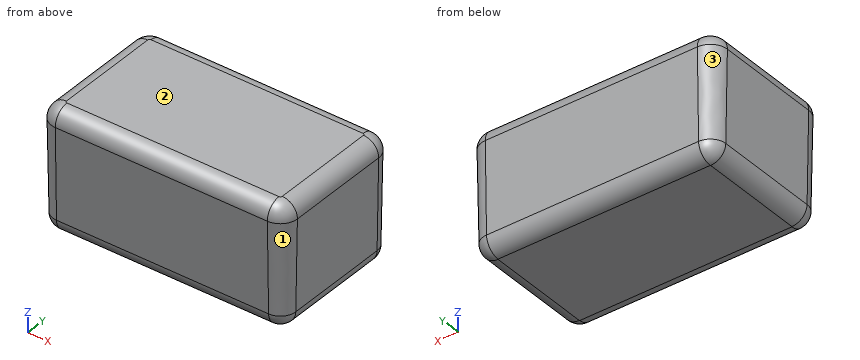
```python
from build123d import *

# Parameters (mm, degrees)
BOSS_EXTRUDE1_DEPTH = 80
DRAFT1_ANGLE        = 1
FILLET1_R           = 10
SHELL2_T            = 2.5


with BuildPart() as part:
    # Sketch1 → Boss-Extrude1 (new body)
    with BuildSketch(Plane.XY):
        with BuildLine():
            Line((-70, 45), (70, 45))
            ThreePointArc((70, 45), (77.071067812, 42.071067812), (80, 35))
            Line((80, 35), (80, -35))
            ThreePointArc((80, -35), (77.071067812, -42.071067812), (70, -45))
            Line((70, -45), (-70, -45))
            ThreePointArc((-70, -45), (-77.071067812, -42.071067812), (-80, -35))
            Line((-80, -35), (-80, 35))
            ThreePointArc((-80, 35), (-77.071067812, 42.071067812), (-70, 45))
        make_face()
    extrude(amount=BOSS_EXTRUDE1_DEPTH)

    # Draft1
    draft1_faces = [part.faces().sort_by_distance(p)[0] for p in [
        (-77.071067812, -42.071067812, 40),
        (-77.071067812, 42.071067812, 40),
        (77.071067812, 42.071067812, 40),
        (77.071067812, -42.071067812, 40),
        (80, 0, 40),
        (0, -45, 40),
        (-80, 0, 40),
        (0, 45, 40),
    ]]
    draft(draft1_faces, Plane(origin=(-70, 35, 0), x_dir=(-1, 0, 0), z_dir=(0, 0, -1)), DRAFT1_ANGLE)

    # Fillet1
    fillet1_edges = [part.edges().sort_by_distance(p)[0] for p in [
        (0, -45, 0),
        (-77.071067812, -42.071067812, 0),
        (-80, 0, 0),
        (-77.071067812, 42.071067812, 0),
        (-78.058475394, -43.058475394, 80),
        (0, -46.396405194, 80),
        (78.058475394, -43.058475394, 80),
        (81.396405194, 0, 80),
        (78.058475394, 43.058475394, 80),
        (0, 46.396405194, 80),
        (-78.058475394, 43.058475394, 80),
        (0, 45, 0),
        (-81.396405194, 0, 80),
        (77.071067812, 42.071067812, 0),
        (80, 0, 0),
        (77.071067812, -42.071067812, 0),
    ]]
    fillet(fillet1_edges, radius=FILLET1_R)

    # Shell2 (no face opened: a closed hollow body)
    add(offset(amount=-SHELL2_T, mode=Mode.PRIVATE), mode=Mode.SUBTRACT)


solid = part.part
```
Geometry: final body of the model. Coordinates: model frame, mm. Face numbers are marked on the shaded views. A direction names the side the tool comes from. Round coordinates to 2 decimals unless told otherwise and drop trailing zeros. Write each loop counter-clockwise with the first axis right and the second up, starting at its lowest first coordinate (ties: lowest second). Pieces come first, ordered by that corner, then holes.
Item 1: Section query B-B (y = -9). Return loops of the section in (x, z).
Item 2: Pin query (flat end, axial travel): P1, Ø4, axis at x = -23.5, z = 45, coming from the +Y side; P2, Ø8, axis at x = -9.5, z = 26, coming from the -Y side; P3, Ø5, axis at y = 30.5, z = 25, coming from the -X side. Return the tip coordinate at first contact, or that it passes through.
Item 3: Set-up query: the marked faces 1, 2 and 3. Return all of +Z, -Z, +X, -X, +Y, -Y with unobstructed straight access to the full face (end or side cutting, diameter ignored); none if empty.
Item 4: Material intervals for L1, parallel to X at y = 2, z = 68; L2, parallel to Z at x = -2, y = -14; L3, parallel to Y at x = 36.5, z = 68, sorted ascending.
Item 5: Section query A-A (x = 61). Return loops of the section in (y, z), plus the area to 3 significant figures.
Completed:
1. outline: (-81.22, 69.83) - (-80.17, 9.83) arc R10 ccw to (-70.17, 0) - (70.17, 0) arc R10 ccw to (80.17, 9.83) - (81.22, 69.83) arc R10 ccw to (71.22, 80) - (-71.22, 80) arc R10 ccw to start; hole (-78.72, 69.87) - (-77.67, 9.87) arc R7.5 ccw to (-70.17, 2.5) - (70.17, 2.5) arc R7.5 ccw to (77.67, 9.87) - (78.72, 69.87) arc R7.5 ccw to (71.22, 77.5) - (-71.22, 77.5) arc R7.5 ccw to start
2. P1: stops at y = 45.82
2. P2: stops at y = -45.52
2. P3: stops at x = -80.48
3. face 1: -Z, +X, -Y
3. face 2: +Z, +X, -X, +Y, -Y
3. face 3: -Z, -X, +Y
4. L1: x = -81.19 to -78.69, 78.69 to 81.19
4. L2: z = 0 to 2.5, 77.5 to 80
4. L3: y = -46.19 to -43.69, 43.69 to 46.19
5. outline: (-46.22, 69.83) - (-45.17, 9.83) arc R10 ccw to (-35.17, 0) - (35.17, 0) arc R10 ccw to (45.17, 9.83) - (46.22, 69.83) arc R10 ccw to (36.22, 80) - (-36.22, 80) arc R10 ccw to start; hole (-43.72, 69.87) - (-42.67, 9.87) arc R7.5 ccw to (-35.17, 2.5) - (35.17, 2.5) arc R7.5 ccw to (42.67, 9.87) - (43.72, 69.87) arc R7.5 ccw to (36.22, 77.5) - (-36.22, 77.5) arc R7.5 ccw to start
5. area: 794 mm2
